Model file for the job. Use its own axes, mm. Give positions to 0.01 mm unless a question says otherwise; leave off trailing zeros. Answer in a Markdown table with one row per item. Add a question column.
Autodesk Inventor part; units mm, degrees
ref_plane "YZ Plane" through (0, 0, 0) normal (1, 0, 0) x (0, 1, 0)
ref_plane "XZ Plane" through (0, 0, 0) normal (0, 1, 0) x (-1, 0, 0)
ref_plane "XY Plane" through (0, 0, 0) normal (0, 0, 1) x (1, 0, 0)
sketch "Sketch1" plane through (0, 0, 0) normal (0, 0, 1) x (1, 0, 0)
  circle A0 centre (0, 0) radius 7.9375
  dimension "d0" = 15.875
extrude "Extrusion1" add sketch "Sketch1" along normal blind 19.05
sketch "Sketch2" plane through (0, 0, 19.05) normal (0, 0, 1) x (1, 0, 0)
  circle A0 centre (0, 0) radius 7.9375
  circle A1 centre (0, 0) radius 11.1125
  dimension "d3" = 3.175
extrude "Extrusion2" add sketch "Sketch2" along normal blind 3.175 contours A0 | A1
chamfer "Chamfer1" distance 0.7937 angle 45 1 edges at (-7.9375, 0, 0)
sketch "Sketch3" plane through (0, 0, 22.225) normal (0, 0, 1) x (1, 0, 0)
  circle A0 centre (0, 0) radius 11.1125
hole "Hole1" at (0, 0, 22.225) direction (0, 0, -1) diameter 12.7 end through all
chamfer "Chamfer2" distance 0.381 angle 45 2 edges at (0, 6.35, 22.225) (0, 6.35, 0)
chamfer "Chamfer3" distance 0.381 angle 45 2 edges at (-11.1125, 0, 22.225) (-11.1125, 0, 19.05)
properties part number "PWTR-0026" material "Bronze, Soft Tin"
Item 1: Wall check: line 1 (Y direction, x = 0, z = 16.5); line 2 (Z direction, x = -4.25, y = 8) (3 decimals); line 3 (Y direction, x = 1.5, z = 16.75). Give the ranges that are in metal, low to high.
Item 2: Pin check, flat tips, straight feed: pin 1 Ø1.5 at (y, z) = (-6, 13) entering from -X; pin 2 Ø3 at (x, z) = (2, 14) entering from -Y; pin 3 Ø7.5 at (x, y) = (0, 0) entering from -Z; pin 4 Ø5 at (y, z) = (4, 14.5) entering from -X. Stop position of each tip, or through.
Item 3: Two-plate mould, pull along X, no slides. Class faces 1 (the cylindrical face through (6.2, 1.38, 10.96)), 2 (the flat face through (5, 5, 22.225)), 3 (the cylindrical face through (10.6, -3.34, 20.62)): pulls with the +X half, pulls with the -X half, needs draft (parallel to the pull), parting line crosses it, or undercut.
Evaluation:
| question | item | result |
|---|---|---|
| 1 | line 1 | y = -7.94 to -6.35, 6.35 to 7.94 |
| 1 | line 2 | z = 19.05 to 22.225 |
| 1 | line 3 | y = -7.79 to -6.17, 6.17 to 7.79 |
| 2 | pin 1 | stops at x = -5.95 |
| 2 | pin 2 | stops at y = -7.92 |
| 2 | pin 3 | passes through |
| 2 | pin 4 | stops at x = -7.79 |
| 3 | face 1 | undercut |
| 3 | face 2 | needs draft |
| 3 | face 3 | parting line crosses it |
